Source: CAD feature listing. Evaluate the final solid. Frame: model axes, mm. Face numbers are marked on the shaded views. Round coordinates to 2 decimals unless told otherwise and drop trailing zeros. Loops run counter-clockwise (first coordinate to the right, second up) from the corner with the lowest first, then second, coordinate; pieces in that order, holes last.
Item 1: Section query B-B on z = 4.65. Return loops of the section in (x, y).
Item 2: Section query A-A on x = 28.2. Return loops of the section in (y, z).
Item 3: Pull-direction query (Z, two-part tool) for the marked faces 1, 2, 3 and 4; classes: released by +Z, released by -Z, zero draft, split by the parting line, or undercut.
Item 4: Section query D-D on z = 26. Return loops of the section in (x, y), then the cut area to 3 significant figures.
Item 5: Ray query, L1, parallel to Z at x = 51.5, y = 4.5; L2, parallel to Y at x = 62, z = 15.5; L3, parallel to X at y = 9.5, z = 11.5. Return the intervals inside material, ascending.
Item 6: Section query C-C on y = 9.5. Return loops of the section in (x, z), then the cut area to 3 significant figures.
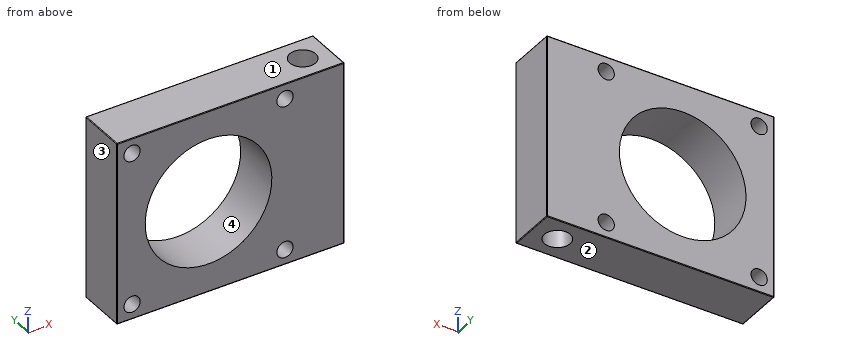
```python
from build123d import *

# Parameters (mm, degrees)
SKETCH1_W           = 70
SKETCH1_H           = 15
SKETCH1_R           = 4
BOSS_EXTRUDE1_DEPTH = 56.4
SKETCH2_R           = 19.5
CUT_EXTRUDE1_DEPTH  = 42.3
SKETCH3_R           = 2.5
CUT_EXTRUDE2_DEPTH  = 92.137039671
FILLET1_R           = 0.2


with BuildPart() as part:
    # Sketch1 → Boss-Extrude1 (new body)
    with BuildSketch(Plane.XY):
        with Locations((35, 7.5)):
            Rectangle(SKETCH1_W, SKETCH1_H)
        with Locations((62, 7.5)):
            Circle(SKETCH1_R, mode=Mode.SUBTRACT)
    extrude(amount=BOSS_EXTRUDE1_DEPTH)

    # Sketch2 → Cut-Extrude1 (cut)
    with BuildSketch(Plane(origin=(0, 15, 0), x_dir=(1, 0, 0), z_dir=(0, 1, 0))):
        with Locations(Location((28.2, -28.2, 0), (0, 0, 270))):
            Circle(SKETCH2_R)
    extrude(amount=-CUT_EXTRUDE1_DEPTH, mode=Mode.SUBTRACT)

    # Sketch3 → Cut-Extrude2 (cut, through all)
    with BuildSketch(Plane(origin=(0, 0, 0), x_dir=(-1, 0, 0), z_dir=(0, -1, 0))):
        with Locations(Location((-51.75, -4.65, 0), (0, 0, 90))):
            Circle(SKETCH3_R)
        with Locations(Location((-4.65, -4.65, 0), (0, 0, 90))):
            Circle(SKETCH3_R)
        with Locations(Location((-4.65, -51.75, 0), (0, 0, 90))):
            Circle(SKETCH3_R)
        with Locations(Location((-51.75, -51.75, 0), (0, 0, 90))):
            Circle(SKETCH3_R)
    extrude(amount=-CUT_EXTRUDE2_DEPTH, mode=Mode.SUBTRACT)

    # Fillet1
    fillet1_edges = [part.edges().sort_by_distance(p)[0] for p in [
        (70, 7.5, 56.4),
        (35, 15, 56.4),
        (0, 7.5, 56.4),
        (35, 15, 0),
        (70, 7.5, 0),
        (35, 0, 0),
        (0, 7.5, 0),
        (35, 0, 56.4),
        (0, 15, 28.2),
        (70, 15, 28.2),
        (70, 0, 28.2),
        (0, 0, 28.2),
    ]]
    fillet(fillet1_edges, radius=FILLET1_R)


solid = part.part
```
Data:
1. outline: (0, 0.2) arc R0.2 ccw to (0.2, 0) - (2.15, 0) - (2.15, 15) - (0.2, 15) arc R0.2 ccw to (0, 14.8) - close; (7.15, 0) - (49.25, 0) - (49.25, 15) - (7.15, 15) - close; (54.25, 0) - (69.8, 0) arc R0.2 ccw to (70, 0.2) - (70, 14.8) arc R0.2 ccw to (69.8, 15) - (54.25, 15) - close; hole circle Ø8 at (62, 7.5)
2. outline: (0, 0.2) arc R0.2 ccw to (0.2, 0) - (14.8, 0) arc R0.2 ccw to (15, 0.2) - (15, 8.7) - (0, 8.7) - close; (0, 47.7) - (15, 47.7) - (15, 56.2) arc R0.2 ccw to (14.8, 56.4) - (0.2, 56.4) arc R0.2 ccw to (0, 56.2) - close
3. face 1: released by +Z
3. face 2: released by -Z
3. face 3: zero draft
3. face 4: undercut
4. outline: (0, 0.2) arc R0.2 ccw to (0.2, 0) - (8.82, 0) - (8.82, 15) - (0.2, 15) arc R0.2 ccw to (0, 14.8) - close; (47.58, 0) - (69.8, 0) arc R0.2 ccw to (70, 0.2) - (70, 14.8) arc R0.2 ccw to (69.8, 15) - (47.58, 15) - close; hole circle Ø8 at (62, 7.5)
4. area: 418 mm2
5. L1: z = 0 to 2.16, 7.14 to 49.26, 54.24 to 56.4
5. L2: y = 0 to 3.5, 11.5 to 15
5. L3: x = 0 to 18.13, 38.27 to 58.54, 65.46 to 70
6. outline: (0, 0.2) arc R0.2 ccw to (0.2, 0) - (58.54, 0) - (58.54, 56.4) - (0.2, 56.4) arc R0.2 ccw to (0, 56.2) - close; (65.46, 0) - (69.8, 0) arc R0.2 ccw to (70, 0.2) - (70, 56.2) arc R0.2 ccw to (69.8, 56.4) - (65.46, 56.4) - close; hole circle Ø5 at (4.65, 4.65); hole circle Ø5 at (4.65, 51.75); hole circle Ø39 at (28.2, 28.2); hole circle Ø5 at (51.75, 4.65); hole circle Ø5 at (51.75, 51.75)
6. area: 2,280 mm2
